```python
from build123d import *

# Parameters (mm, degrees)
F0_W     = 8
F0_H     = 3
F1_DEPTH = 5
F0_W_2   = 7
F0_H_2   = 4
F2_DEPTH = 40
F0_W_3   = 5
F0_H_3   = 10
F3_DEPTH = 3
F0_W_4   = 20
F0_H_4   = 12
F4_DEPTH = 2
F5_DEPTH = 1


with BuildPart() as f1:
    # F0 (on Top) → F1 (new body)
    with BuildSketch(Plane.XY):
        with Locations((-15.1580379307, 9.4352371395)):
            Rectangle(F0_W, F0_H)
    extrude(amount=F1_DEPTH)



with BuildPart() as f2:
    # F0 (on Top) → F2 (new body)
    with BuildSketch(Plane.XY):
        with Locations((-14.7853907049, 2.9733350016)):
            Rectangle(F0_W_2, F0_H_2)
    extrude(amount=F2_DEPTH)


with BuildPart() as f3:
    # F0 (on Top) → F3 (new body)
    with BuildSketch(Plane.XY):
        with Locations((-4.0641951468, 6.3341652229)):
            Rectangle(F0_W_3, F0_H_3)
    extrude(amount=F3_DEPTH)


with BuildPart() as f1_1:
    add(f1.part)

    add(f2.part)  # F4 merges F2

    add(f3.part)  # F4 merges F3
    # F0 (on Top) → F4 (join)
    with BuildSketch(Plane.XY):
        with Locations((-10, 6)):
            Rectangle(F0_W_4, F0_H_4)
        with Locations((-14.7853907049, 2.9733350016)):
            Rectangle(F0_W_2, F0_H_2, mode=Mode.SUBTRACT)
        with Locations((-15.1580379307, 9.4352371395)):
            Rectangle(F0_W, F0_H, mode=Mode.SUBTRACT)
        with Locations((-4.0641951468, 6.3341652229)):
            Rectangle(F0_W_3, F0_H_3, mode=Mode.SUBTRACT)
    extrude(amount=-F4_DEPTH)

    # F0 (on Top) → F5 (join)
    with BuildSketch(Plane.XY):
        with Locations((-14.7853907049, 2.9733350016)):
            Rectangle(F0_W_2, F0_H_2)
        with Locations((-15.1580379307, 9.4352371395)):
            Rectangle(F0_W, F0_H)
        with Locations((-4.0641951468, 6.3341652229)):
            Rectangle(F0_W_3, F0_H_3)
    extrude(amount=-F5_DEPTH)


solid = f1_1.part
```
Geometry: final body of the model. Coordinates: model frame, mm. A direction names the side the tool comes from. Coordinates: 2 decimals unless noted, no trailing zeros. Order: outer loops, then holes, each group sorted by start corner. A loop starts at its lowest first (then second) coordinate and runs counter-clockwise, first axis right, second up. Notation, with made-up numbers: (0.5, -30) -> (40.5, -30) arc R27 ccw to (40.5, -13) -> close; hole circle Ø3 at (31, 76.25). An arc over 180 degrees is marked (long way). Write item = value, one per line.
(1) Cut plane D-D on z = 23. Return loops of the section in (x, y), plus the area to 3 significant figures.
Solved:
outline = (-18.29, 0.97) -> (-11.29, 0.97) -> (-11.29, 4.97) -> (-18.29, 4.97) -> close
area = 28.0 mm²
(2) Line query: line 1 (X direction, y = 4.5, z = 2); line 2 (Z direction, x = -8, y = 6.25); line 3 (Y direction, x = -11.75, z = 15). Output: solid intervals per line, ascending.
Solved:
line_1 = -18.29 to -11.29, -6.56 to -1.56
line_2 = -2 to 0
line_3 = 0.97 to 4.97
(3) Pull-direction query (X, two-part tool) for faces 5 (the flat face through (-1.564, 6, 1)), 6 (the flat face through (-10, 6, -2)), 7 (the flat face through (-18.285, 2.9, -1.5)); classes: pulls with the +X half, pulls with the -X half, needs draft (parallel to the pull), parting line crosses it, or undercut.
Solved:
face_5 = pulls with the +X half
face_6 = needs draft
face_7 = undercut
(4) Cut plane B-B on x = -3.5. Return loops of the section in (y, z).
Solved:
outline = (0, -2) -> (1.33, -2) -> (1.33, -1) -> (11.33, -1) -> (11.33, -2) -> (12, -2) -> (12, 0) -> (11.33, 0) -> (11.33, 3) -> (1.33, 3) -> (1.33, 0) -> (0, 0) -> close
(5) Access query for faces 1 (the flat face through (-4.1, 1.334, -1.5)), 2 (the flat face through (-15, 9, 5)), 3 (the flat face through (-4, 6, 3)), 4 (the flat face through (-19.158, 9, 2)). Directions: +Z, -Z, +X, -X, +Y, -Y. A direction counts if a zero-diameter tool reaches every point of the face in a straight line with its end or side. Return the directions, or none.
Solved:
face_1 = -Z
face_2 = +Z, +X, -X, +Y
face_3 = +Z, +X, +Y, -Y
face_4 = +Z, -X, +Y, -Y
(6) Pin query (flat end, axial travel): pin 1 Ø7.5 at (x, z) = (-16.5, 22) entering from -Y; pin 2 Ø12 at (x, z) = (-8.5, 18) entering from +Y; pin 3 Ø4 at (y, z) = (4.5, 17.5) entering from +X. Return the tip coordinate at first contact, or that it passes through.
Solved:
pin_1 = 0.97
pin_2 = 4.97
pin_3 = -11.29
(7) Cut plane C-C on x = -14.25. Return loops of the section in (y, z), plus the area to 3 significant figures.
Solved:
outline = (0, -2) -> (0.97, -2) -> (0.97, -1) -> (4.97, -1) -> (4.97, -2) -> (7.94, -2) -> (7.94, -1) -> (10.94, -1) -> (10.94, -2) -> (12, -2) -> (12, 0) -> (10.94, 0) -> (10.94, 5) -> (7.94, 5) -> (7.94, 0) -> (4.97, 0) -> (4.97, 40) -> (0.97, 40) -> (0.97, 0) -> (0, 0) -> close
area = 192 mm²
(8) Cut plane A-A on y = 3.25. Return loops of the section in (x, z).
Solved:
outline = (-20, -2) -> (-18.29, -2) -> (-18.29, -1) -> (-11.29, -1) -> (-11.29, -2) -> (-6.56, -2) -> (-6.56, -1) -> (-1.56, -1) -> (-1.56, -2) -> (0, -2) -> (0, 0) -> (-1.56, 0) -> (-1.56, 3) -> (-6.56, 3) -> (-6.56, 0) -> (-11.29, 0) -> (-11.29, 40) -> (-18.29, 40) -> (-18.29, 0) -> (-20, 0) -> close
